CAD build for the part. Positions are in the model's coordinates, mm. Face numbers are marked on the shaded views. A direction names the side the tool comes from. Coordinates: 2 decimals unless noted, no trailing zeros. Order: outer loops, then holes, each group sorted by start corner. A loop starts at its lowest first (then second) coordinate and runs counter-clockwise, first axis right, second up. Notation, with made-up numbers: (89.25, 18.25) - (117.25, 18.25) arc R10 cw to (117.25, 34.25) - close; hole circle Ø8 at (-8, 34). An arc over 180 degrees is marked (long way). Write each question's results on one line, items separated by ' | '. Start each with the question number.
Q1. Band-saw the part on C-C, the plane x = -9.5. Write the cut outline in (y, z) (3 decimals).
Q2. Band-saw the part on B-B, the plane y = -14.5. Write the cut outline in (x, z) (3 decimals).
Q3. Pull direction Z, two halves, no side cores. Call the marked faces 3, 4 and 5: released by +Z, released by -Z, zero draft, split by the parting line, or undercut.
Q4. Wall check: probe 1 along Z at (x, y) = (-4.25, 18.5) (3 decimals); probe 2 along Y at (x, z) = (-11.5, 18.5); probe 3 along X at (y, z) = (9, 11) (3 decimals). Give the ranges that are in metal, low to high.
Q5. Band-saw the part on D-D, the plane y = 4.5. Write the cut outline in (x, z) (3 decimals).
Q6. Which spindle directions (+Z, -Z, +X, -X, +Y, -Y) get a long thin tool onto all of the face, cutting with end or side? Do the marked faces 1 and 2. Say none if no direction does.
Q7. Pin check, flat tip, straight feed: P1, Ø10, axis at y = 2, z = 10, coming from the -X side (3 decimals). Stop position of the tip, or through.
Q8. Band-saw the part on A-A, the plane x = -4. Write the cut outline in (y, z) (3 decimals).
```python
from build123d import *

# Parameters (mm, degrees)
SKETCH1_W               = 25.4
SKETCH1_H               = 50.8
BOSS_EXTRUDE1_DEPTH     = 3.175
SKETCH4_W               = 6.35
SKETCH4_H               = 50.8
BOSS_EXTRUDE2_DEPTH     = 12.7
SKETCH5_W               = 9.525
SKETCH5_H               = 50.8
BOSS_EXTRUDE3_DEPTH     = 25.4
F_1_4_CLEARANCE_HOLE1_D = 7.14248
FILLET1_R               = 3.175


with BuildPart() as part:
    # Sketch1 → Boss-Extrude1 (new, symmetric)
    with BuildSketch(Plane(origin=(0, 0, 0), x_dir=(0, 0, -1), z_dir=(1, 0, 0))):
        Rectangle(SKETCH1_W, SKETCH1_H)
    extrude(amount=BOSS_EXTRUDE1_DEPTH, both=True)

    # Sketch4 → Boss-Extrude2 (add)
    with BuildSketch(Plane.XY.offset(12.7)):
        Rectangle(SKETCH4_W, SKETCH4_H)
    boss_extrude2 = extrude(amount=BOSS_EXTRUDE2_DEPTH)

    # Sketch5 → Boss-Extrude3 (add)
    with BuildSketch(Plane(origin=(3.175, 0, 0), x_dir=(0, 0, -1), z_dir=(1, 0, 0))):
        with Locations((-20.6375, 0)):
            Rectangle(SKETCH5_W, SKETCH5_H)
    boss_extrude3 = extrude(amount=-BOSS_EXTRUDE3_DEPTH)

    # Mirror1: Boss-Extrude2, Boss-Extrude3 across plane
    add(boss_extrude2.mirror(Plane.XY))
    add(boss_extrude3.mirror(Plane.XY))

    # 1/4 Clearance Hole1 (through all)
    with Locations(Plane(origin=(-9.866844114, 16.191031899, 25.4), x_dir=(1, 0, 0), z_dir=(0, 0, 1))):
        with Locations((0, 0), (-0.677264826, -32.232776497)):
            Hole(F_1_4_CLEARANCE_HOLE1_D / 2)

    # Fillet1
    fillet1_edges = [part.edges().sort_by_distance(p)[0] for p in [
        (-22.225, 25.4, 20.6375),
        (-22.225, -25.4, 20.6375),
        (-22.225, -25.4, -20.6375),
        (-22.225, 25.4, -20.6375),
    ]]
    fillet(fillet1_edges, radius=FILLET1_R)


solid = part.part
```
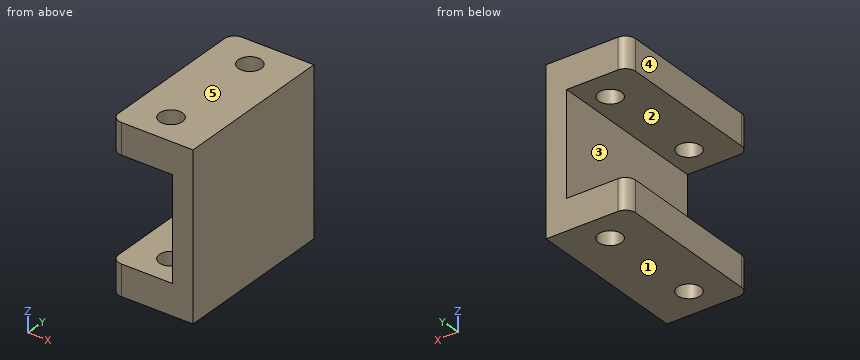
Results below:
1) outline: (-25.4, -25.4) - (-19.457, -25.4) - (-19.457, -15.875) - (-25.4, -15.875) - close; (-25.4, 15.875) - (-19.457, 15.875) - (-19.457, 25.4) - (-25.4, 25.4) - close; (-12.627, -25.4) - (12.639, -25.4) - (12.639, -15.875) - (-12.627, -15.875) - close; (-12.627, 15.875) - (12.639, 15.875) - (12.639, 25.4) - (-12.627, 25.4) - close; (19.743, -25.4) - (25.4, -25.4) - (25.4, -15.875) - (19.743, -15.875) - close; (19.743, 15.875) - (25.4, 15.875) - (25.4, 25.4) - (19.743, 25.4) - close
2) outline: (-22.225, -25.4) - (-13.765, -25.4) - (-13.765, -15.875) - (-22.225, -15.875) - close; (-22.225, 15.875) - (-13.765, 15.875) - (-13.765, 25.4) - (-22.225, 25.4) - close; (-7.323, -25.4) - (3.175, -25.4) - (3.175, 25.4) - (-7.323, 25.4) - (-7.323, 15.875) - (-3.175, 15.875) - (-3.175, -15.875) - (-7.323, -15.875) - close
3) face 3: undercut | face 4: zero draft | face 5: released by +Z
4) probe 1: z = -25.4 to -15.875, 15.875 to 25.4 | probe 2: y = -25.4 to -19.48, -12.6 to 13.02, 19.37 to 25.4 | probe 3: x = -3.175 to 3.175
5) outline: (-22.225, -25.4) - (3.175, -25.4) - (3.175, 25.4) - (-22.225, 25.4) - (-22.225, 15.875) - (-3.175, 15.875) - (-3.175, -15.875) - (-22.225, -15.875) - close
6) face 1: -Z, +X, -X, +Y, -Y | face 2: -X, +Y, -Y
7) P1: stops at x = -3.175
8) outline: (-25.4, -25.4) - (25.4, -25.4) - (25.4, -15.875) - (-25.4, -15.875) - close; (-25.4, 15.875) - (25.4, 15.875) - (25.4, 25.4) - (-25.4, 25.4) - close
